For this review, take the finished solid that the model builds, in its own axes (mm). Face numbers are marked on the shaded views. A direction names the side the tool comes from. Coordinates: 2 decimals unless noted, no trailing zeros. Loops run counter-clockwise (first coordinate to the right, second up) from the corner with the lowest first, then second, coordinate; pieces in that order, holes last. Notation, with made-up numbers: M -9.5,10.5 L 41.5,10.5 A17 ccw 41.5,20.5 Z; hole C -26.5,60.5 d1. An arc over 180 degrees is marked long. Write each question's results on one line, items separated by ' | '. Start each with the question number.
```python
from build123d import *

# Parameters (mm, degrees)
Y_KSEKLIK_EKSTR_ZYON2_DEPTH = 50
Y_KSEKLIK_EKSTR_ZYON3_DEPTH = 5
IZIM3_W                     = 51.443502464
IZIM3_H                     = 5
KES_EKSTR_ZYON1_DEPTH       = 15
IZIM4_W                     = 15
IZIM4_H                     = 4
KES_EKSTR_ZYON2_DEPTH       = 90
RADYUS2_R                   = 10
RADYUS3_R                   = 10
KES_EKSTR_ZYON3_REACH       = 96.271
IZIM5_R                     = 3.5
KES_EKSTR_ZYON4_DEPTH       = 103.312244464
KES_EKSTR_ZYON4_DEPTH_BACK  = 103.312244464
IZIM6_R                     = 5


with BuildPart() as part:
    # Çizim1 → Yükseklik-Ekstrüzyon2 (new body)
    with BuildSketch(Plane.XY):
        Polygon((-7.114525921, 27.60391198), (7.885474079, 27.60391198), (7.885474079, -22.39608802), (-82.114525921, -22.39608802), (-82.114525921, -7.39608802), (-7.114525921, -7.39608802), align=None)
    extrude(amount=Y_KSEKLIK_EKSTR_ZYON2_DEPTH)

    # Çizim2 → Yükseklik-Ekstrüzyon3 (add)
    with BuildSketch(Plane(origin=(0, -7.39608802, 0), x_dir=(1, 0, 0), z_dir=(0, 1, 0))):
        with BuildLine():
            Line((-7.114525921, 0), (-30.671023457, 0))
            Line((-30.671023457, 0), (-30.671023457, -5))
            ThreePointArc((-30.671023457, -5), (-10.671023457, -25), (-30.671023457, -45))
            Line((-30.671023457, -45), (-30.671023457, -50))
            Line((-30.671023457, -50), (-7.114525921, -50))
            Line((-7.114525921, -50), (-7.114525921, 0))
        make_face()
    extrude(amount=Y_KSEKLIK_EKSTR_ZYON3_DEPTH)

    # Çizim3 → Kes-Ekstrüzyon1 (cut)
    with BuildSketch(Plane(origin=(0, -7.39608802, 0), x_dir=(1, 0, 0), z_dir=(0, 1, 0))):
        with Locations((-56.392774689, -2.5)):
            Rectangle(IZIM3_W, IZIM3_H)
        with Locations((-56.392774689, -47.5)):
            Rectangle(IZIM3_W, IZIM3_H)
    extrude(amount=-KES_EKSTR_ZYON1_DEPTH, mode=Mode.SUBTRACT)

    # Çizim4 → Kes-Ekstrüzyon2 (cut)
    with BuildSketch(Plane.ZY.offset(82.114525921)):
        with Locations((25, -20.39608802)):
            Rectangle(IZIM4_W, IZIM4_H)
    extrude(amount=-KES_EKSTR_ZYON2_DEPTH, mode=Mode.SUBTRACT)

    # Radyus2
    radyus2_edges = [part.edges().sort_by_distance(p)[0] for p in [
        (0.385474079, 27.60391198, 0),
    ]]
    fillet(radyus2_edges, radius=RADYUS2_R)

    # Radyus3
    radyus3_edges = [part.edges().sort_by_distance(p)[0] for p in [
        (0.385474079, 27.60391198, 50),
    ]]
    fillet(radyus3_edges, radius=RADYUS3_R)

    # Çizim5 → Kes-Ekstrüzyon3 (cut, up to next)
    with BuildSketch(Plane.ZY.offset(7.114525921), mode=Mode.PRIVATE) as kes_ekstr_zyon3_sk1:
        with Locations(Location((10, 17.60391198, 0), (0, 0, 270))):
            Circle(IZIM5_R)
    kes_ekstr_zyon3_tool1 = extrude(kes_ekstr_zyon3_sk1.sketch, amount=-KES_EKSTR_ZYON3_REACH, mode=Mode.PRIVATE) & part.part
    # Çizim5 → Kes-Ekstrüzyon3 (cut, up to next)
    with BuildSketch(Plane.ZY.offset(7.114525921), mode=Mode.PRIVATE) as kes_ekstr_zyon3_sk2:
        with Locations(Location((40, 17.60391198, 0), (0, 0, 270))):
            Circle(IZIM5_R)
    kes_ekstr_zyon3_tool2 = extrude(kes_ekstr_zyon3_sk2.sketch, amount=-KES_EKSTR_ZYON3_REACH, mode=Mode.PRIVATE) & part.part
    add(kes_ekstr_zyon3_tool1.solids().sort_by_distance((-7.114526, 17.603912, 10))[0], mode=Mode.SUBTRACT)
    add(kes_ekstr_zyon3_tool2.solids().sort_by_distance((-7.114526, 17.603912, 40))[0], mode=Mode.SUBTRACT)

    # Çizim6 → Kes-Ekstrüzyon4 (cut, two sides: drawn at the far end of the back side and taken through both)
    with BuildSketch(Plane(origin=(0, -7.39608802, 0), x_dir=(1, 0, 0), z_dir=(0, 1, 0)).offset(-KES_EKSTR_ZYON4_DEPTH_BACK)):
        with Locations((-30.671023457, -25)):
            Circle(IZIM6_R)
        with BuildLine():
            Line((-72.114525921, -20), (-52.114525921, -20))
            ThreePointArc((-52.114525921, -20), (-47.114525921, -25), (-52.114525921, -30))
            Line((-52.114525921, -30), (-72.114525921, -30))
            ThreePointArc((-72.114525921, -30), (-77.114525921, -25), (-72.114525921, -20))
        make_face()
    extrude(amount=KES_EKSTR_ZYON4_DEPTH + KES_EKSTR_ZYON4_DEPTH_BACK, mode=Mode.SUBTRACT)


solid = part.part
```
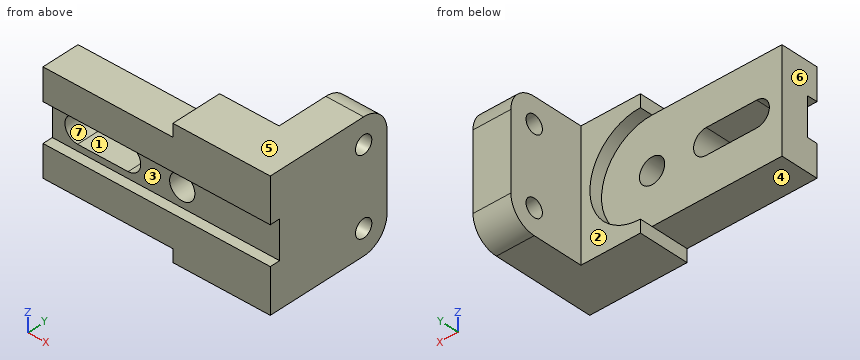
Q1. Insertion check: P1, Ø1.5, axis at y = -10.5, z = 47, coming from the -X side; P2, Ø9, axis at x = -30.67, z = 25, coming from the -Y side; P3, Ø3.5, axis at x = -60, y = -15.5, coming from the +Z side; P4, Ø9, axis at x = -64, y = -12.5, coming from the -Z side. Each pin has a flat end and moves straight along its axis. Give the tip position at first contact, or say it passes through.
Q2. For the marked faces 1, 2, 3 and 4, list the 3-axis set-ups (+Z, -Z, +X, -X, +Y, -Y) from which the entire face can be reached by the end or side of a thin tool; tool diameter is ignored.
Q3. Take a section at D-D, the plane z = 38. Give the boundary of the cut face in (x, y).
Q4. Take a section at B-B, the plane x = -70. Give the boundary of the cut face in (y, z).
Q5. To check wall thickness, follow line 1 along Y through (x, z) = (-38, 33); line 2 along Y through (x, z) = (-13.5, 12.5); line 3 along X through (y, z) = (2, 32.5). State the ranges of each line that lie inside material, in increasing order.
Q6. Take a section at C-C, the plane x = -8.5. Give the boundary of the cut face in (y, z), then the cut area to 3 significant figures.
Q7. The part is to be moulded in two halves that separate along X. For the marked faces 5, 6 and 7, say which applies: pulls with the +X half, pulls with the -X half, needs draft (parallel to the pull), parting line crosses it, or undercut.
Q8. Take a section at A-A, the plane z = 25. Give the boundary of the cut face in (x, y), then the cut area to 3 significant figures.
Results:
1) P1: x = -30.67 | P2: through | P3: z = 45 | P4: z = 5
2) face 1: +Y, -Y | face 2: +Z, -Z, -X, +Y | face 3: +X, -X, -Y | face 4: -Z, -X, +Y, -Y
3) outline: M -82.11,-22.4 L 7.89,-22.4 L 7.89,14.73 L -7.11,14.73 L -7.11,-2.4 L -15.47,-2.4 L -15.47,-7.4 L -82.11,-7.4 Z; M -7.11,20.48 L 7.89,20.48 L 7.89,27.6 L -7.11,27.6 Z
4) outline: M -22.4,5 L -7.4,5 L -7.4,20 L -18.4,20 L -18.4,17.5 L -22.4,17.5 Z; M -22.4,32.5 L -18.4,32.5 L -18.4,30 L -7.4,30 L -7.4,45 L -22.4,45 Z
5) line 1: -22.4 to -7.4 | line 2: -22.4 to -2.4 | line 3: -7.11 to 7.89
6) outline: M -22.4,0 L -2.4,0 L -2.4,50 L -22.4,50 L -22.4,32.5 L -18.4,32.5 L -18.4,17.5 L -22.4,17.5 Z | area: 940 mm^2
7) face 5: needs draft | face 6: pulls with the -X half | face 7: undercut
8) outline: M -82.11,-18.4 L -77.11,-18.4 L -77.11,-7.4 L -82.11,-7.4 Z; M -47.11,-18.4 L -35.67,-18.4 L -35.67,-7.4 L -47.11,-7.4 Z; M -25.67,-18.4 L 7.89,-18.4 L 7.89,27.6 L -7.11,27.6 L -7.11,-2.4 L -10.67,-2.4 L -10.67,-7.4 L -25.67,-7.4 Z | area: 1,090 mm^2
